Can you work these out from the model? Positions are in its coordinate system, mm. Coordinates: 2 decimals unless noted, no trailing zeros. Loops run counter-clockwise (first coordinate to the right, second up) from the corner with the lowest first, then second, coordinate; pieces in that order, holes last. Notation, with made-up numbers: (69, 9) - (85, 9) arc R12 cw to (85, 31) - close; hole circle Ø1 at (63.5, 60). An arc over 180 degrees is marked (long way). Put each result on its own line as item: value. Start each with the question number.
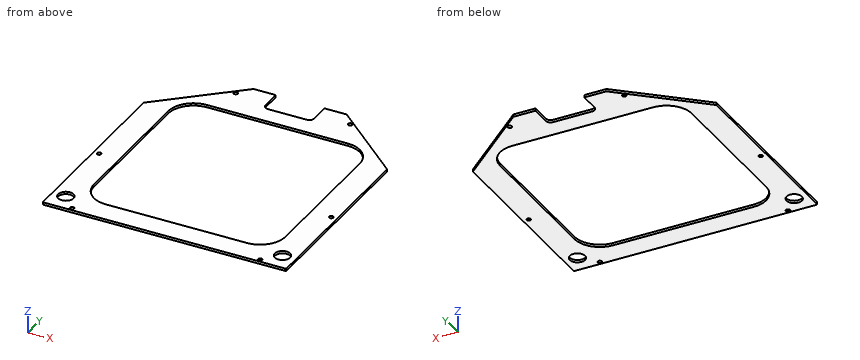
from build123d import *

# Parameters (mm, degrees)
BOSS_EXTRUDE1_DEPTH        = 1.6002
F_2_CLEARANCE_HOLE1_D      = 2.7051
SKETCH8_W                  = 31.75
SKETCH8_H                  = 15.875
CUT_EXTRUDE3_DEPTH         = 2.6002
FILLET1_R                  = 3.175
F_10_0_10_DIAMETER_HOLE1_D = 10


with BuildPart() as part:
    # Sketch2 → Boss-Extrude1 (new body)
    with BuildSketch(Plane.XY.offset(1.5875)):
        with BuildLine():
            Line((70.711408136, 21.697450137), (10.568555904, 21.697450137))
            ThreePointArc((10.568555904, 21.697450137), (10.389483229, 21.664841533), (10.233399988, 21.571201994))
            Line((10.233399988, 21.571201994), (-38.276423867, -21.017595986))
            ThreePointArc((-38.276423867, -21.017595986), (-38.404043925, -21.189818895), (-38.449267951, -21.399347884))
            Line((-38.449267951, -21.399347884), (-38.449267951, -145.180549937))
            ThreePointArc((-38.449267951, -145.180549937), (-38.300478171, -145.539760241), (-37.941267867, -145.688549937))
            Line((-37.941267867, -145.688549937), (119.221232133, -145.688549937))
            ThreePointArc((119.221232133, -145.688549937), (119.580442454, -145.53976015), (119.729232133, -145.18054983))
            Line((119.729232133, -145.18054983), (119.729232133, -21.399347777))
            ThreePointArc((119.729232133, -21.399347777), (119.684008101, -21.189818753), (119.556387965, -21.017595879))
            Line((119.556387965, -21.017595879), (71.046564052, 21.571202036))
            ThreePointArc((71.046564052, 21.571202036), (70.890480797, 21.664841536), (70.711408136, 21.697450137))
        make_face()
        with BuildLine():
            Line((102.869982113, -114.451909481), (102.869982113, -22.874190224))
            ThreePointArc((102.869982113, -22.874190224), (98.05448357, -11.248548333), (86.428841679, -6.433049852))
            Line((86.428841679, -6.433049852), (-5.148877578, -6.433049852))
            ThreePointArc((-5.148877578, -6.433049852), (-16.774519469, -11.248548395), (-21.59001795, -22.874190286))
            Line((-21.59001795, -22.874190286), (-21.59001795, -114.451909543))
            ThreePointArc((-21.59001795, -114.451909543), (-16.774519407, -126.077551434), (-5.148877516, -130.893049915))
            Line((-5.148877516, -130.893049915), (86.428841741, -130.893049915))
            ThreePointArc((86.428841741, -130.893049915), (98.054483632, -126.077551372), (102.869982113, -114.451909481))
        make_face(mode=Mode.SUBTRACT)
    extrude(amount=BOSS_EXTRUDE1_DEPTH)

    # #2 Clearance Hole1 (through all)
    with Locations(Plane.XY.offset(3.1877)):
        with Locations((3.4816648, 12.855075079), (77.798299252, 12.855075129), (-34.763097208, -82.95054975), (116.04306139, -82.950549647), (101.758732132, -143.593049842), (-20.478767868, -143.593049925)):
            Hole(F_2_CLEARANCE_HOLE1_D / 2)

    # Sketch8 → Cut-Extrude3 (cut, through all)
    with BuildSketch(Plane.XY.offset(3.1877)):
        with Locations((40.63998202, 13.759950137)):
            Rectangle(SKETCH8_W, SKETCH8_H)
    extrude(amount=-CUT_EXTRUDE3_DEPTH, mode=Mode.SUBTRACT)

    # Fillet1
    fillet1_edges = [part.edges().sort_by_distance(p)[0] for p in [
        (56.51498202, 5.822450137, 2.3876),
        (24.76498202, 5.822450137, 2.3876),
    ]]
    fillet(fillet1_edges, radius=FILLET1_R)

    # Ø10.0 (10) Diameter Hole1 (through all)
    with Locations(Plane(origin=(0, 0, 1.5875), x_dir=(-1, 0, 0), z_dir=(0, 0, -1))):
        with Locations((-111.045602766, -133.661649696), (29.765638361, -133.661649887)):
            Hole(F_10_0_10_DIAMETER_HOLE1_D / 2)


solid = part.part
Q1. Please list where these lines run through material, in increasing order: line 1 along X through (y, z) = (-85.5, 2); line 2 along Y through (x, z) = (67, 2.1); line 3 along Y through (x, z) = (29, 3.1). Write a range as [from, to].
Q2. I want a section at C-C on z = 2.9. Count the separate pieces of the cut face and the enclosed holes in it, and give its area (3 significant figures).
Q3. I want a section at A-A on x = 30. List the corners of the cut face in (y, z) for me, and give its area (3 significant figures).
Q4. Will these pins go through, and if not, where does the flat tip stop? pin 1 (6 mm diameter, centred on x = 111.05, y = -133.66, fed in from +Z); pin 2 (0.8 mm diameter, centred on y = 13, z = 2, fed in from -X).
Q5. I want a section at B-B on y = -104. List the corners of the cut face in (x, z) for me, and give its area (3 significant figures).
Calculated:
1. line 1: [-38.45, -21.59], [102.87, 119.73]
1. line 2: [-145.69, -130.89], [-6.43, 21.7]
1. line 3: [-145.69, -130.89], [-6.43, 5.82]
2. separate pieces: 1
2. enclosed holes: 9
2. area: 8,430 mm2
3. outline: (-145.69, 1.59) - (-130.89, 1.59) - (-130.89, 3.19) - (-145.69, 3.19) - close; (-6.43, 1.59) - (5.82, 1.59) - (5.82, 3.19) - (-6.43, 3.19) - close
3. area: 43.3 mm2
4. pin 1: through
4. pin 2: x = 0.01
5. outline: (-38.45, 1.59) - (-21.59, 1.59) - (-21.59, 3.19) - (-38.45, 3.19) - close; (102.87, 1.59) - (119.73, 1.59) - (119.73, 3.19) - (102.87, 3.19) - close
5. area: 54.0 mm2
